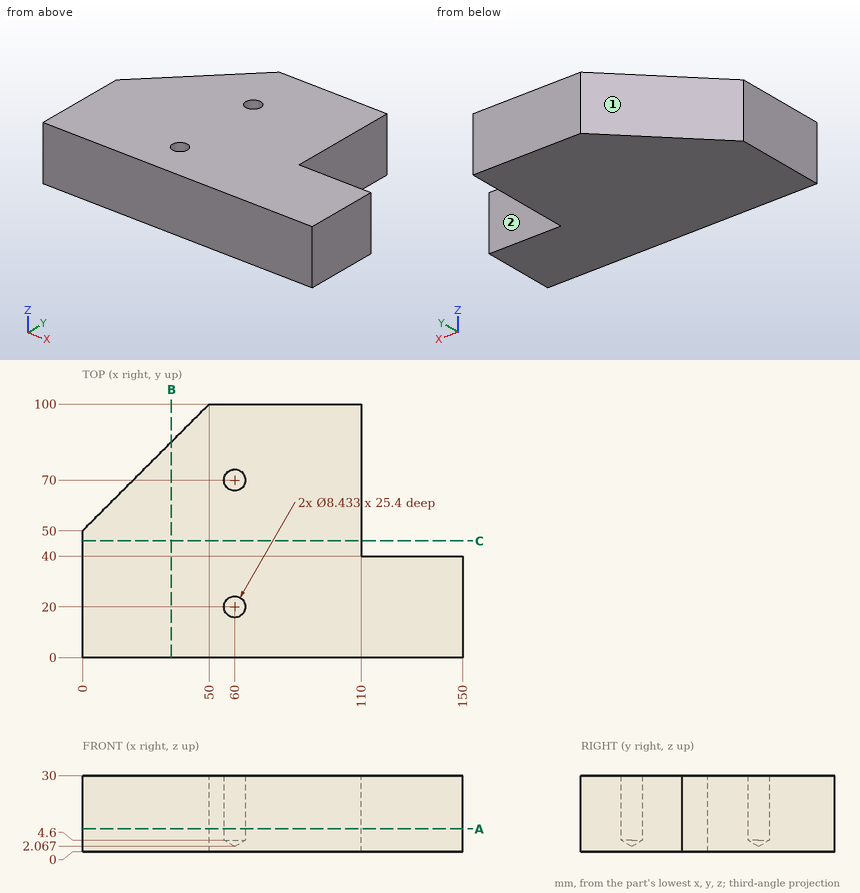
Geometry: see drawing. Coordinates: mm, zero at the bounding-box minimum. A direction names the side the tool comes from. Give positions to 0.01 mm unless a question says otherwise; leave off trailing zeros. Loops run counter-clockwise (first coordinate to the right, second up) from the corner with the lowest first, then second, coordinate; pieces in that order, holes last. Notation, with made-up numbers: (-17, 62) -> (38, 62) arc R24 cw to (38, 99) -> close; hole circle Ø1 at (52.5, -28). An arc over 180 degrees is marked (long way). Answer as a JSON object with one key per item and string values. Group by question number.
Item 1: Cut plane B-B, the plane x = 35. Return the cut outline in (y, z), and give its area (3 significant figures).
Item 2: Pin query (flat end, axial travel): P1, Ø3, axis at x = 46.5, z = 17, coming from the +Y side; P2, Ø9, axis at x = 129.5, z = 19.5, coming from the +Y side; P3, Ø10, axis at y = 86.5, z = 18, coming from the +X side. Return the tip coordinate at first contact, or that it passes through.
Item 3: Cut plane A-A, the plane z = 9. Return the cut outline in (x, y).
Item 4: Cut plane C-C, the plane y = 46. Return the cut outline in (x, z).
Item 5: Line query: probe 1 along Y at (x, z) = (60, 9.75); probe 2 along X at (y, z) = (20, 11.25); probe 3 along X at (y, z) = (70, 23.5) (1 decimal). Output: solid intervals per line, ascending.
Item 6: Reachability of the marked faces 1 and 2 from +Z, -Z, +X, -X, +Y, -Y: full face, straight path, thin tool, end or side. Return the list, or none.
Checks:
{
 "1": {"outline": "(0, 0) -> (85, 0) -> (85, 30) -> (0, 30) -> close", "area": "2,550 mm²"},
 "2": {"P1": "stops at y = 98", "P2": "stops at y = 40", "P3": "stops at x = 110"},
 "3": {"outline": "(0, 0) -> (150, 0) -> (150, 40) -> (110, 40) -> (110, 100) -> (50, 100) -> (0, 50) -> close; hole circle Ø8.43 at (60, 20); hole circle Ø8.43 at (60, 70)"},
 "4": {"outline": "(0, 0) -> (110, 0) -> (110, 30) -> (0, 30) -> close"},
 "5": {"probe 1": "y = 0 to 15.78, 24.22 to 65.78, 74.22 to 100", "probe 2": "x = 0 to 55.78, 64.22 to 150", "probe 3": "x = 20 to 55.8, 64.2 to 110"},
 "6": {"face 1": "+Z, -Z, -X, +Y", "face 2": "+Z, -Z, +X, +Y"}
}
